from build123d import *

# Parameters (mm, degrees)
SKETCH001_W  = 2.5
SKETCH001_H  = 5
PAD001_DEPTH = 0.5
SKETCH002_W  = 2.5
SKETCH002_H  = 5
PAD002_DEPTH = 0.5
SKETCH_W     = 12.5
SKETCH_H     = 12.5
PAD_DEPTH    = 5.5
FILLET_R     = 1.5
SKETCH003_R  = 5
POCKET_DEPTH = 3
FILLET001_R  = 0.3


with BuildPart() as body001:
    # Sketch001 → Pad001 (new body)
    with BuildSketch(Plane.XY):
        with Locations((-4.75, 0)):
            Rectangle(SKETCH001_W, SKETCH001_H)
    extrude(amount=PAD001_DEPTH)


with BuildPart() as body002:
    # Sketch002 → Pad002 (new body)
    with BuildSketch(Plane.XY):
        with Locations((4.75, 0)):
            Rectangle(SKETCH002_W, SKETCH002_H)
    extrude(amount=PAD002_DEPTH)


with BuildPart() as fusion:
    # Sketch → Pad (new body)
    with BuildSketch(Plane.XY):
        Rectangle(SKETCH_W, SKETCH_H)
    extrude(amount=PAD_DEPTH)

    # Fillet
    fillet_edges = [fusion.edges().sort_by_distance(p)[0] for p in [
        (-6.25, -6.25, 2.75),
        (6.25, -6.25, 2.75),
        (-6.25, 6.25, 2.75),
        (6.25, 6.25, 2.75),
    ]]
    fillet(fillet_edges, radius=FILLET_R)

    # Sketch003 (on Face5 of Fillet) → Pocket (cut)
    with BuildSketch(Plane.XY.offset(5.5)):
        with BuildLine():
            ThreePointArc((-4.678742, 2.891258), (-5.5, 0), (-4.678742, -2.891258))
            ThreePointArc((-4.678742, -2.891258), (-4.919239, -4.919239), (-2.891258, -4.678742))
            ThreePointArc((-2.891258, -4.678742), (0, -5.5), (2.891258, -4.678742))
            ThreePointArc((2.891258, -4.678742), (4.919239, -4.919239), (4.678742, -2.891258))
            ThreePointArc((4.678742, -2.891258), (5.5, 0), (4.678742, 2.891258))
            ThreePointArc((4.678742, 2.891258), (4.919239, 4.919239), (2.891258, 4.678742))
            ThreePointArc((2.891258, 4.678742), (0, 5.5), (-2.891258, 4.678742))
            ThreePointArc((-2.891258, 4.678742), (-4.919239, 4.919239), (-4.678742, 2.891258))
        make_face()
        Circle(SKETCH003_R, mode=Mode.SUBTRACT)
    extrude(amount=-POCKET_DEPTH, mode=Mode.SUBTRACT)

    # Fillet001
    fillet001_edges = [fusion.edges().sort_by_distance(p)[0] for p in [
        (-5, 0, 5.5),
    ]]
    fillet(fillet001_edges, radius=FILLET001_R)


with BuildPart() as fusion_1:
    # Body placement: moved
    add(fusion.part.moved(Location((0, 0, 0.5))))

    # Fusion: union Body001, Body002
    add(body001.part)
    add(body002.part)


solid = fusion_1.part
Here's how the part is built. I have some questions about the finished solid (model axes, mm). A direction names the side the tool comes from. Coordinates: 2 decimals unless noted, no trailing zeros. Order: outer loops, then holes, each group sorted by start corner. A loop starts at its lowest first (then second) coordinate and runs counter-clockwise, first axis right, second up. Notation, with made-up numbers: M 44,16.5 L 91,16.5 A18 ccw 91,37.5 Z; hole C 1.25,-25 d7. An arc over 180 degrees is marked long. Answer as CSV lines item,"result". Start each with the question number.
1. For pin 1 (0.6 mm diameter, centred on x = 5.5, z = 0, fed in from +Y); pin 2 (6 mm diameter, centred on x = 2.5, y = -4, fed in from -Z); pin 3 (2.5 mm diameter, centred on x = 4, y = -4, fed in from -Z), each with a flat end and sliding along its axis, tell me the tip position at first contact or that it passes through.
2. On a 3-axis mill with a long thin cutter (end or side, diameter ignored), from which of +Z, -Z, +X, -X, +Y, -Y can I reach the whole of each face in a straight line? I mean faces 4 (the flat face through (0, -6.25, 3)), 5 (the cylindrical face through (0, -5.5, 4.5)). Say none if no direction works.
3. I want a section at A-A, the plane z = 3.3. Write out the boundary of the cut face in (x, y).
4. We'd pull the mould along Y, two halves only. Please class faces 1 (the flat face through (0, 0, 6)), 2 (the flat face through (0, 6.25, 3)), 3 (the cylindrical face through (5.5, 0, 4.5)): released by +Y, released by -Y, zero draft, split by the parting line, or undercut.
5. I want a section at C-C, the plane y = 5.75. Write out the boundary of the cut face in (x, z), and give its area (3 significant figures).
6. I need wall thicknesses on line 1 (X direction, y = 1, z = 5.55); line 2 (X direction, y = -4, z = 4.95). Which ranges of each line are inside material? Lowest first, please. Write a range as [from, to].
7. I want a section at B-B, the plane x = 0. Write out the boundary of the cut face in (y, z).
Recorded:
1,pin 1,"stops at y = 2.5"
1,pin 2,"stops at z = 0"
1,pin 3,"stops at z = 0.5"
2,face 4,"+Z, -Z, +X, -X, -Y"
2,face 5,"+Z"
3,outline,"M -6.25,-4.75 A1.5 ccw -4.75,-6.25 L 4.75,-6.25 A1.5 ccw 6.25,-4.75 L 6.25,4.75 A1.5 ccw 4.75,6.25 L -4.75,6.25 A1.5 ccw -6.25,4.75 Z; C 0,0 d10; hole M -4.68,-2.89 A1.3 ccw long -2.89,-4.68 A5.5 ccw 2.89,-4.68 A1.3 ccw long 4.68,-2.89 A5.5 ccw 4.68,2.89 A1.3 ccw long 2.89,4.68 A5.5 ccw -2.89,4.68 A1.3 ccw long -4.68,2.89 A5.5 ccw Z"
4,face 1,"zero draft"
4,face 2,"released by +Y"
4,face 3,"undercut"
5,outline,"M -5.87,0.5 L 5.87,0.5 L 5.87,6 L -5.87,6 Z"
5,area,"64.5 mm2"
6,line 1,"x = [-6.25, -5.41], [-4.9, 4.9], [5.41, 6.25]"
6,line 2,"x = [-6.25, -5.3], [-3, 3], [5.3, 6.25]"
7,outline,"M -6.25,0.5 L 6.25,0.5 L 6.25,6 L 5.5,6 L 5.5,3 L 5,3 L 5,5.7 A0.3 ccw 4.7,6 L -4.7,6 A0.3 ccw -5,5.7 L -5,3 L -5.5,3 L -5.5,6 L -6.25,6 Z"
